```python
from build123d import *

# Parameters (mm, degrees)
F0_R      = 9.398
F1_DEPTH  = 15.875
F4_R      = 7.62
F4_R_2    = 7.3025
F5_DEPTH  = 1.5875
F6_R      = 7.3025
F7_DEPTH  = 2.032
F8_W      = 5.08
F8_H      = 5.08
F9_DEPTH  = 6.35
F10_W     = 4.064
F10_H     = 4.7625
F10_R     = 1.23825
F11_DEPTH = 2.032


with BuildPart() as f1:
    # F0 (on Top) → F1 (new body)
    with BuildSketch(Plane.XY):
        Circle(F0_R)
    extrude(amount=-F1_DEPTH)

    # F2 (on Front) → F3 (revolve)
    with BuildSketch(Plane.XZ):
        Polygon((0, 1.5875), (0, 0), (10.922, 0), (8.73125, 1.5875), align=None)
    revolve(axis=Axis((0, 0, 0.79375), (0, 0, -1)))

    # F4 (on face) → F5 (cut)
    with BuildSketch(Plane.XY.offset(1.5875)):
        Circle(F4_R)
        Circle(F4_R_2, mode=Mode.SUBTRACT)
    extrude(amount=-F5_DEPTH, mode=Mode.SUBTRACT)

    # F6 (on face) → F7 (join)
    with BuildSketch(Plane(origin=(0, 0, -15.875), x_dir=(1, 0, 0), z_dir=(0, 0, -1))):
        Circle(F6_R)
    extrude(amount=F7_DEPTH)

    # F8 (on face) → F9 (join)
    with BuildSketch(Plane(origin=(0, 0, -17.907), x_dir=(1, 0, 0), z_dir=(0, 0, -1))):
        Rectangle(F8_W, F8_H)
    extrude(amount=F9_DEPTH)

    # F10 (on Front) → F11 (join, symmetric)
    with BuildSketch(Plane.XZ):
        with Locations((-4.572, -20.28825)):
            Rectangle(F10_W, F10_H)
        with Locations((-4.572, -19.6215)):
            Circle(F10_R, mode=Mode.SUBTRACT)
        with Locations((4.572, -20.28825)):
            Rectangle(F10_W, F10_H)
        with Locations((4.572, -19.6215)):
            Circle(F10_R, mode=Mode.SUBTRACT)
    extrude(amount=F11_DEPTH, both=True)


solid = f1.part
```
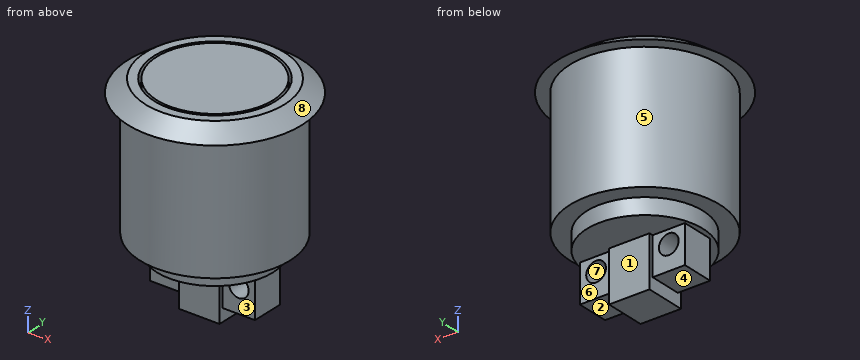
CAD build for the part. Positions are in the model's coordinates, mm. Face numbers are marked on the shaded views. A direction names the side the tool comes from. Round coordinates to 2 decimals unless told otherwise and drop trailing zeros. Write each loop counter-clockwise with the first axis right and the second up, starting at its lowest first coordinate (ties: lowest second). Pieces come first, ordered by that corner, then holes.
Item 1: Band-saw the part on B-B on y = 0. Give the number of separate pieces and of enclosed holes in the cut face, then the cut area to 3 significant figures.
Filled in:
separate pieces: 1
enclosed holes: 2
area: 420 mm2
Item 2: Drill centre lines: L1, parallel to Z at x = 4.5, y = 0; L2, parallel to Z at x = -5.5, y = -4.5; L3, parallel to Y at x = 2.75, z = -21. Where is each one in solid material? Low to high.
Filled in:
L1: z = -22.67 to -20.86, -18.39 to 1.59
L2: z = -17.91 to 1.59
L3: y = -2.03 to 2.03
Item 3: Band-saw the part on D-D on z = -2.5. Write the cut outline in (x, y).
Filled in:
outline: circle Ø18.8 at (0, 0)
Item 4: Band-saw the part on C-C on z = -17. Write the cut outline in (x, y) (1 decimal).
Filled in:
outline: circle Ø14.6 at (0, 0)
Item 5: Drop flat-ended pins along their axis: pin 1 Ø12 at (x, z) = (7.5, -7) entering from -Y; pin 2 Ø3 at (y, z) = (-7.5, -14) entering from +X; pin 3 Ø1 at (y, z) = (-8, -10.5) entering from -X. Give the stop position or say it passes through.
Filled in:
pin 1: stops at y = -9.28
pin 2: stops at x = 7.23
pin 3: stops at x = -5.66
Item 6: Tool access for the marked faces 1, 2, 3, 4 and 5: list every direction of +Z, -Z, +X, -X, +Y, -Y with a clear straight run to the whole face (end or side of a thin tool).
Filled in:
face 1: -Z, +X, -X, +Y
face 2: -Z, +X, +Y, -Y
face 3: -Z, +X, -Y
face 4: -Z, -X, +Y, -Y
face 5: -Z
Item 7: Mould opens along X. For the marked faces 6, 7 and 8 say: released by +X, released by -X, zero draft, split by the parting line, or undercut.
Filled in:
face 6: zero draft
face 7: undercut
face 8: split by the parting line
